from build123d import *

# Parameters (mm, degrees)
SKETCH1_W                = 159
SKETCH1_H                = 101
SKETCH1_R                = 1.5
MAIN_BOARD_DEPTH         = 1.6
SKETCH2_W                = 50.87
SKETCH2_H                = 8.71
CONNECTOR_DEPTH          = 9.24
SKETCH3_W                = 1.6
SKETCH3_H                = 112.2
CONNECTOR_BOARD_DEPTH    = 52.04
SKETCH4_R                = 7.5
CAN_CONNECTOR_DEPTH      = 28
SKETCH5_R                = 8.8
MAIN_LV_CONNECTOR_DEPTH  = 21
SKETCH6_R                = 3.93
SERIAL_CONNECTOR_DEPTH   = 18.5
SKETCH7_R                = 8.775
FEEDBACK_CONNECTOR_DEPTH = 14.5


with BuildPart() as part:
    # Sketch1 → Main Board (new body)
    with BuildSketch(Plane(origin=(0, 0, 0), x_dir=(1, 0, 0), z_dir=(0, 1, 0))):
        Rectangle(SKETCH1_W, SKETCH1_H)
        with Locations((-25, 45.5)):
            Circle(SKETCH1_R, mode=Mode.SUBTRACT)
        with Locations((30.5, 40.5)):
            Circle(SKETCH1_R, mode=Mode.SUBTRACT)
        with Locations((-74.5, -44.5)):
            Circle(SKETCH1_R, mode=Mode.SUBTRACT)
        with Locations((60.5, -44.5)):
            Circle(SKETCH1_R, mode=Mode.SUBTRACT)
    extrude(amount=MAIN_BOARD_DEPTH)

    # Sketch2 → Connector (add)
    with BuildSketch(Plane(origin=(0, 1.6, 0), x_dir=(1, 0, 0), z_dir=(0, 1, 0))):
        with Locations((-54.065, 45.145)):
            Rectangle(SKETCH2_W, SKETCH2_H)
    extrude(amount=CONNECTOR_DEPTH)

    # Sketch3 → Connector Board (add)
    with BuildSketch(Plane(origin=(0, 1.6, 0), x_dir=(1, 0, 0), z_dir=(0, 1, 0))):
        with Locations((74.7, 0.4)):
            Rectangle(SKETCH3_W, SKETCH3_H)
    extrude(amount=CONNECTOR_BOARD_DEPTH)

    # Sketch4 → CAN Connector (add)
    with BuildSketch(Plane(origin=(75.5, 0, 0), x_dir=(0, 0, -1), z_dir=(1, 0, 0))):
        with Locations((45.5, 41.64)):
            Circle(SKETCH4_R)
    extrude(amount=CAN_CONNECTOR_DEPTH)

    # Sketch5 → Main LV Connector (add)
    with BuildSketch(Plane(origin=(75.5, 0, 0), x_dir=(0, 0, -1), z_dir=(1, 0, 0))):
        with Locations((22.5, 41.64)):
            Circle(SKETCH5_R)
    extrude(amount=MAIN_LV_CONNECTOR_DEPTH)

    # Sketch6 → Serial Connector (add)
    with BuildSketch(Plane(origin=(75.5, 0, 0), x_dir=(0, 0, -1), z_dir=(1, 0, 0))):
        with Locations((1.5, 41.64)):
            Circle(SKETCH6_R)
    extrude(amount=SERIAL_CONNECTOR_DEPTH)

    # Sketch7 → Feedback Connector (add)
    with BuildSketch(Plane(origin=(75.5, 0, 0), x_dir=(0, 0, -1), z_dir=(1, 0, 0))):
        with Locations((-18.5, 41.64)):
            Circle(SKETCH7_R)
    extrude(amount=FEEDBACK_CONNECTOR_DEPTH)


solid = part.part
Here's how the part is built. I have some questions about the finished solid (model axes, mm). A direction names the side the tool comes from. Give positions to 0.01 mm unless a question says otherwise; leave off trailing zeros. Order: outer loops, then holes, each group sorted by start corner. A loop starts at its lowest first (then second) coordinate and runs counter-clockwise, first axis right, second up. Notation, with made-up numbers: (58.5, 9.5) -> (101.5, 9.5) arc R27 ccw to (101.5, 27.5) -> close; hole circle Ø9 at (-39, -23.5). An arc over 180 degrees is marked (long way). One line per item, written item: value. Start each with the question number.
1. Imagine slicing it at B-B, the plane x = 83. List the corners of the cut face in (y, z) for me (3 decimals), plus the area to 3 significant figures.
2. I need wall thicknesses on probe 1 along X at (y, z) = (0.5, 44.5); probe 2 along Z at (x, y) = (-25, 1.2); probe 3 along X at (y, z) = (1.1, -40.5). Which ranges of each line are inside material? Lowest first, please. Write a range as from..to.
3. Imagine slicing it at C-C, the plane z = -34.5. List the corners of the cut face in (x, y) for me.
4. We'd pull the mould along Z, two halves only. Please class faces 6 (the face through (-54, 6, -40.79)), 7 (the face through (89.304, 43.893, -52.654)), 8 (the face through (96.5, 42, -22)): released by +Z, released by -Z, zero draft, split by the parting line, or undercut.
5. For faces 1 (the face through (-28.63, 6, -45)), 2 (the face through (-54, 6, -49.5)), 3 (the face through (77, 1.6, -1)), 4 (the face through (82.65, 44.28, 10.13)), 5 (the face through (-54, 10.84, -45)), which set-ups out of +Z, -Z, +X, -X, +Y, -Y let a thin tool reach every point of the face, with its end or its side?
6. Imagine slicing it at D-D, the plane x = -62. List the corners of the cut face in (y, z) for me.
7. Imagine slicing it at A-A, the plane y = 9. List the corners of the cut face in (x, z) for me.
8. Will these pins go through, and if not, where does the flat tip stop? pin 1 Ø4.5 at (y, z) = (7.5, -43.5) entering from +X; pin 2 Ø15.5 at (y, z) = (28.5, -19.5) entering from +X; pin 3 Ø1.5 at (x, z) = (7.5, -39) entering from +Y; pin 4 Ø5 at (x, y) = (81, 28) entering from -Z.
Values follow:
1. outline: circle Ø17.6 at (41.64, -22.5); circle Ø17.55 at (41.64, 18.5); circle Ø15 at (41.64, -45.5); circle Ø7.86 at (41.64, -1.5)
1. area: 710 mm2
2. probe 1: x = -79.5..-76, -73..59, 62..79.5
2. probe 2: z = -50.5..-47, -44..50.5
2. probe 3: x = -79.5..29, 32..79.5
3. outline: (-79.5, 0) -> (79.5, 0) -> (79.5, 1.6) -> (75.5, 1.6) -> (75.5, 53.64) -> (73.9, 53.64) -> (73.9, 1.6) -> (-79.5, 1.6) -> close
4. face 6: released by +Z
4. face 7: undercut
4. face 8: zero draft
5. face 1: +Z, -Z, +Y
5. face 2: -Z, -X, +Y
5. face 3: +Z, -Z, +X
5. face 4: +X
5. face 5: +Z, -Z, -X, +Y
6. outline: (0, -50.5) -> (1.6, -50.5) -> (1.6, -49.5) -> (10.84, -49.5) -> (10.84, -40.79) -> (1.6, -40.79) -> (1.6, 50.5) -> (0, 50.5) -> close
7. outline: (-79.5, -49.5) -> (-28.63, -49.5) -> (-28.63, -40.79) -> (-79.5, -40.79) -> close; (73.9, -56.5) -> (75.5, -56.5) -> (75.5, 55.7) -> (73.9, 55.7) -> close
8. pin 1: stops at x = 75.5
8. pin 2: stops at x = 96.5
8. pin 3: stops at y = 1.6
8. pin 4: passes through
